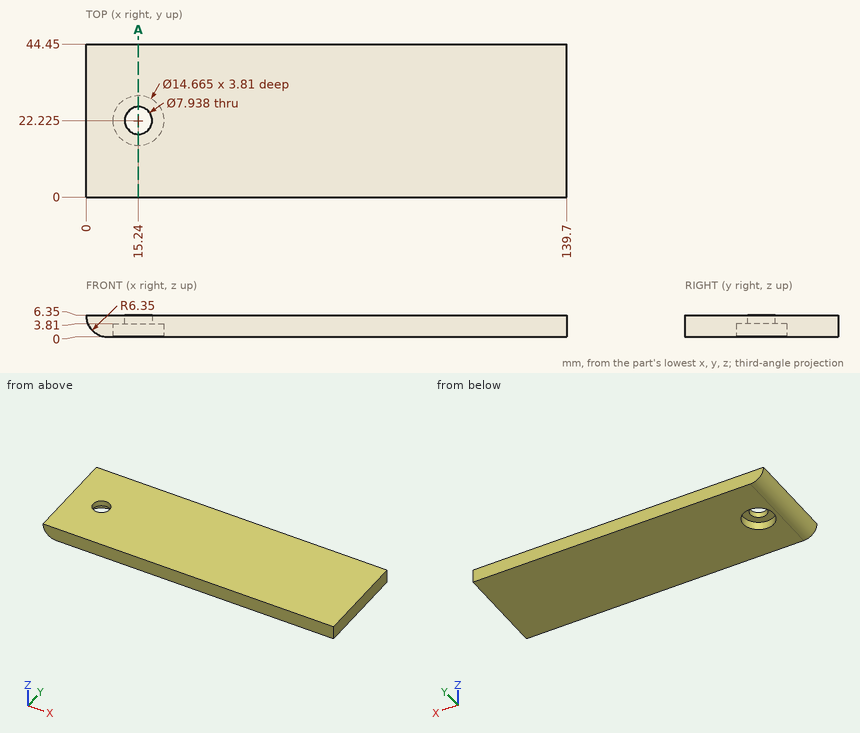
Here's the drawing with two shaded views (mm, measured from the low corner). I have some questions. Give positions to 0.01 mm unless a question says otherwise; leave off trailing zeros. Loops run counter-clockwise (first coordinate to the right, second up) from the corner with the lowest first, then second, coordinate; pieces in that order, holes last. Notation, with made-up numbers: (80.5, 17) - (100.5, 17) arc R30 ccw to (100.5, 49) - close; hole circle Ø8 at (-1, 69.5). An arc over 180 degrees is marked (long way). One line per item, written item: value.
(1) If we section it at A-A, the plane x = 15.24: List the corners of the cut face in (y, z) for me, plus the area to 3 significant figures.
Verdict:
outline: (0, 0) - (14.89, 0) - (14.89, 3.81) - (18.26, 3.81) - (18.26, 6.35) - (0, 6.35) - close; (26.19, 3.81) - (29.56, 3.81) - (29.56, 0) - (44.45, 0) - (44.45, 6.35) - (26.19, 6.35) - close
area: 206 mm^2
(2) I'm going to push a flat-ended pin straight in: pin 1 (4.5 mm diameter, centred on x = 14, y = 25.5, fed in from -Z). Where does the tip first touch, or does it pass through?
Verdict:
pin 1: z = 3.81
(3) I need wall thicknesses on line 1 along Y through (x, z) = (15.5, 3.5); line 2 along Y through (x, z) = (15.24, 5.35); line 3 along X through (y, z) = (16.5, 1) (1 decimal). Which ranges of each line are inside material? Lowest first, please.
Verdict:
line 1: 0 to 14.9, 29.55 to 44.45
line 2: 0 to 18.26, 26.19 to 44.45
line 3: 2.9 to 10.7, 19.8 to 139.7
